Geometry check sheet. Reference: the model listing, model coordinates, mm. A direction names the side the tool comes from. Give positions to 0.01 mm unless a question says otherwise; leave off trailing zeros. Order: outer loops, then holes, each group sorted by start corner. A loop starts at its lowest first (then second) coordinate and runs counter-clockwise, first axis right, second up. Notation, with made-up numbers: M -32.5,28 L -5.5,28 A25 ccw -5.5,58 Z; hole C 78,-36.75 d8. An arc over 180 degrees is marked long. One line per question, with ' | ' between items. Start each with the question number.
from build123d import *

# Parameters (mm, degrees)
SKETCH1_R           = 11.9
SKETCH1_R_2         = 9.9
BOSS_EXTRUDE3_DEPTH = 15
SKETCH4_R           = 9.9
BOSS_EXTRUDE4_DEPTH = 5.1
BOSS_EXTRUDE8_START = -3
SKETCH12_R          = 19
SKETCH12_R_2        = 11.9
BOSS_EXTRUDE8_DEPTH = 3
SKETCH14_R          = 1.755
CUT_EXTRUDE4_DEPTH  = 3


with BuildPart() as part:
    # Sketch1 → Boss-Extrude3 (new body)
    with BuildSketch(Plane(origin=(0, 0, 0), x_dir=(1, 0, 0), z_dir=(0, 1, 0))):
        with Locations(Location((0, 0, 0), (0, 0, 270))):
            Circle(SKETCH1_R)
        with Locations(Location((0, 0, 0), (0, 0, 270))):
            Circle(SKETCH1_R_2, mode=Mode.SUBTRACT)
    extrude(amount=BOSS_EXTRUDE3_DEPTH)

    # Sketch4 → Boss-Extrude4 (add)
    with BuildSketch(Plane.XZ):
        with Locations(Location((0, 0, 0), (0, 0, 270))):
            Circle(SKETCH4_R)
    extrude(amount=-BOSS_EXTRUDE4_DEPTH)

    # Sketch7 → Cut-Revolve2 (revolve, cut)
    with BuildSketch(Plane(origin=(0, 0, 0), x_dir=(0, 0, -1), z_dir=(1, 0, 0))):
        with BuildLine():
            Line((0, 15), (0, -4.8))
            ThreePointArc((0, -4.8), (9.9, 5.1), (0, 15))
        make_face()
    revolve(axis=Axis((0, 15, 0), (0, -1, 0)), mode=Mode.SUBTRACT)

    # Sketch12 → Boss-Extrude8 (add)
    with BuildSketch(Plane(origin=(0, 15, 0), x_dir=(1, 0, 0), z_dir=(0, 1, 0)).offset(BOSS_EXTRUDE8_START)):
        with Locations(Location((0, 0, 0), (0, 0, 270))):
            Circle(SKETCH12_R)
        with Locations(Location((0, 0, 0), (0, 0, 270))):
            Circle(SKETCH12_R_2, mode=Mode.SUBTRACT)
    extrude(amount=BOSS_EXTRUDE8_DEPTH)

    # Sketch14 → Cut-Extrude4 (cut)
    with BuildSketch(Plane(origin=(0, 15, 0), x_dir=(1, 0, 0), z_dir=(0, 1, 0))):
        with Locations(Location((0, 15.15, 0), (0, 0, 270))):
            Circle(SKETCH14_R)
        with Locations(Location((-15.15, 0, 0), (0, 0, 270))):
            Circle(SKETCH14_R)
        with Locations(Location((0, -15.15, 0), (0, 0, 270))):
            Circle(SKETCH14_R)
        with Locations(Location((15.15, 0, 0), (0, 0, 270))):
            Circle(SKETCH14_R)
    extrude(amount=-CUT_EXTRUDE4_DEPTH, mode=Mode.SUBTRACT)


solid = part.part
Item 1: Depth check by flat-ended pin: pin 1 (6 mm diameter, centred on y = 3, z = 8, fed in from +X); pin 2 (5.5 mm diameter, centred on x = 0, z = 15.15, fed in from +Y); pin 3 (2 mm diameter, centred on x = -10.5, z = -14.5, fed in from -Y); pin 4 (3 mm diameter, centred on x = 15.15, z = 0, fed in from +Y). Enter the tip coordinate at first touch or a pass-through.
Item 2: Set-up check for faces 4 (the cylindrical face through (-11.56, 13.48, -15.08)), 5 (the flat face through (9, 12, -9)), 6 (the cylindrical face through (2.974, 9.981, 9.443)): record each of +Z, -Z, +X, -X, +Y, -Y from which the full face is reachable in a straight line by a thin tool's end or side.
Item 3: Cross-section at A-A, the plane x = -15.15. Record the cut outline in (y, z) (3 decimals).
Item 4: Cross-section at B-B, the plane z = -3.5. Record the cut outline in (x, y), plus the area to 3 significant figures.
Item 5: Cross-section at C-C, the plane x = 0. Record the cut outline in (y, z) (3 decimals).
Item 6: Mould release check, pull along X, two halves, no side actions. Record for faces 1 (the flat face through (-8, 15, 8)), 2 (the cylindrical face through (3.57, 5.92, 11.35)), 3 (the cylindrical face through (0.527, 13.521, -13.476)): released by +X, released by -X, zero draft, split by the parting line, or undercut.
Item 7: Material ranges on line 1 along X through (y, z) = (12.7, 0) (3 decimals); line 2 along X through (y, z) = (10.75, 0); line 3 along Y through (x, z) = (-14.5, 8.5), recorded low to high.
Item 8: Cross-section at D-D, the plane y = 13.5. Record the cut outline in (x, z) (3 decimals), plus the area to 3 significant figures.
Outcome:
1) pin 1: stops at x = 10.8 | pin 2: stops at y = 15 | pin 3: stops at y = 12 | pin 4: passes through
2) face 4: +Y, -Y | face 5: -Y | face 6: +Y
3) outline: M 12,-11.466 L 15,-11.466 L 15,-1.755 L 12,-1.755 Z; M 12,1.755 L 15,1.755 L 15,11.466 L 12,11.466 Z
4) outline: M -18.67,12 L -11.37,12 L -11.37,0 L -7.73,0 A9.26 cw -9.26,5.1 L -9.26,15 L -18.67,15 Z; M 7.73,0 L 11.37,0 L 11.37,12 L 18.67,12 L 18.67,15 L 9.26,15 L 9.26,5.1 A9.26 cw Z | area: 112 mm²
5) outline: M 0,-11.9 L 12,-11.9 L 12,-13.395 L 15,-13.395 L 15,-9.9 L 5.1,-9.9 A9.9 cw 0,-8.485 Z; M 0,8.485 A9.9 cw 5.1,9.9 L 15,9.9 L 15,13.395 L 12,13.395 L 12,11.9 L 0,11.9 Z; M 12,-19 L 15,-19 L 15,-16.905 L 12,-16.905 Z; M 12,16.905 L 15,16.905 L 15,19 L 12,19 Z
6) face 1: zero draft | face 2: split by the parting line | face 3: undercut
7) line 1: x = -19 to -16.905, -13.395 to -9.9, 9.9 to 13.395, 16.905 to 19 | line 2: x = -11.9 to -9.9, 9.9 to 11.9 | line 3: y = 12 to 15
8) outline: C 0,0 d38; hole C -15.15,0 d3.51; hole C 0,0 d19.8; hole C 0,-15.15 d3.51; hole C 0,15.15 d3.51; hole C 15.15,0 d3.51 | area: 788 mm²
